Part print with two shaded views. Sizes in mm from the minimum x, y, z corner. Coordinates: 2 decimals unless noted, no trailing zeros. Loops run counter-clockwise (first coordinate to the right, second up) from the corner with the lowest first, then second, coordinate; pieces in that order, holes last.
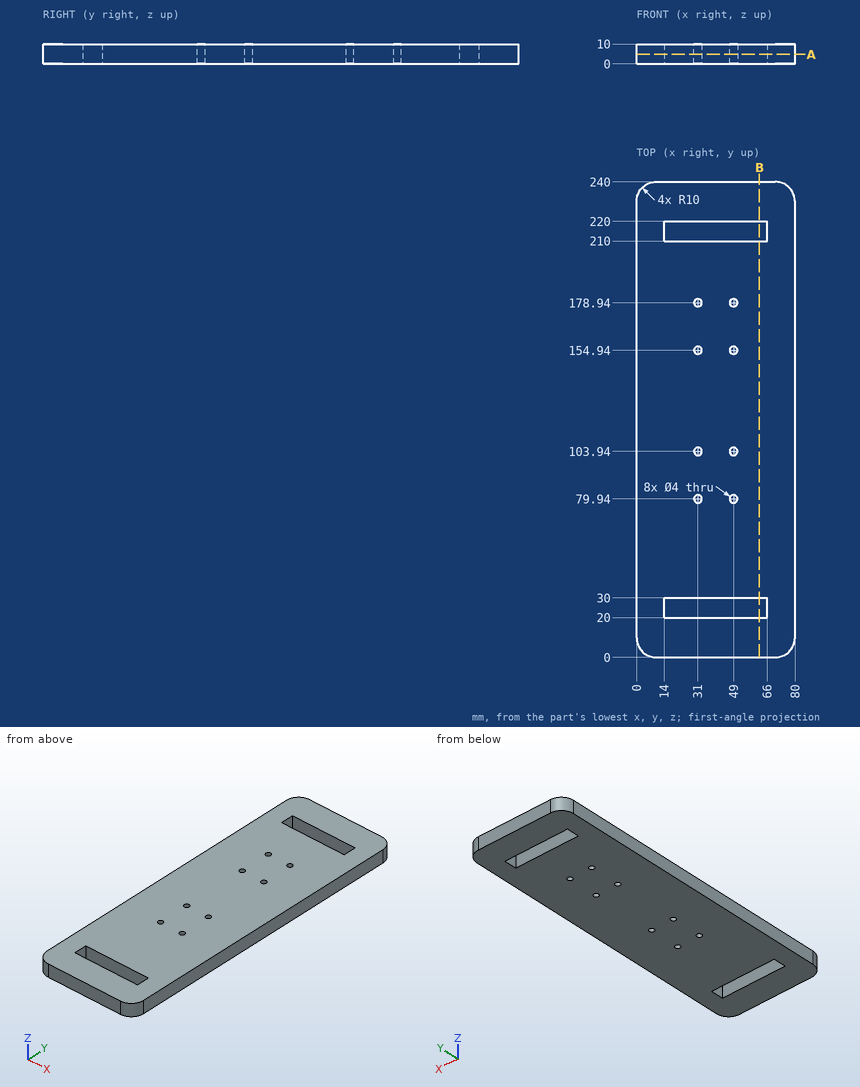
Q1. Slice it at B-B (x = 62). List the corners of the cut face in (y, z).
Answers:
outline: (0, 0) - (20, 0) - (20, 10) - (0, 10) - close; (30, 0) - (210, 0) - (210, 10) - (30, 10) - close; (220, 0) - (240, 0) - (240, 10) - (220, 10) - close
Q2. Drill centre lines: line 1 (Y direction, x = 37, z = 6.5); line 2 (X direction, y = 178.94, z = 7.75); line 3 (Y direction, x = 77, z = 4). Where is each one in solid material? Low to high.
Answers:
line 1: y = 0 to 20, 30 to 210, 220 to 240
line 2: x = 0 to 29, 33 to 47, 51 to 80
line 3: y = 2.86 to 237.14
Q3. Slice it at A-A (z = 4.75). Count the separate pieces of the cut face and the enclosed holes in it, and give its area (3 significant figures).
Answers:
separate pieces: 1
enclosed holes: 10
area: 18,000 mm2
